Build history of the part. All positions in model axes, mm. Face numbers are marked on the shaded views. A direction names the side the tool comes from. Give positions to 0.01 mm unless a question says otherwise; leave off trailing zeros. Write each loop counter-clockwise with the first axis right and the second up, starting at its lowest first coordinate (ties: lowest second). Pieces come first, ordered by that corner, then holes. Notation, with made-up numbers: (3.5, 21.5) - (23.5, 21.5) arc R20 cw to (23.5, 59.5) - close; hole circle Ø4 at (23.5, 49). An arc over 180 degrees is marked (long way). Use one line per item in the form item = value. Start each with the question number.
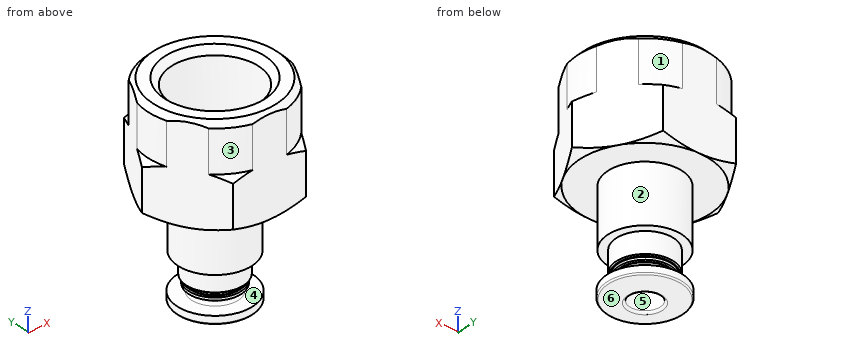
Autodesk Inventor part; units mm, degrees
ref_plane "ANBAU_STD_XY" through (0, 0, 0) normal (0, 0, -1) x (1, 0, 0)
ref_plane "ANBAU_STD_YZ" through (0, 0, 0) normal (1, 0, 0) x (0, -1, 0)
ref_plane "ANBAU_STD_ZX" through (0, 0, 0) normal (0, -1, 0) x (0, 0, -1)
sketch "Sketch_1" plane through (0, 0, 0) normal (1, 0, 0) x (0, 1, 0)
  line L0 (0, -26.9) -> (0, 0)
  line L1 (0, 0) -> (10.2, 0)
  line L2 (10.2, 0) -> (10.2, -20.6)
  line L3 (10.2, -20.6) -> (3.75, -20.6)
  line L4 (3.75, -20.6) -> (3.75, -23.35)
  line L5 (3.75, -23.35) -> (3.6, -23.5)
  line L6 (3.6, -23.5) -> (3.45, -23.5)
  line L7 (3.45, -23.5) -> (3.45, -23.85)
  line L8 (3.45, -23.85) -> (3.3, -24)
  line L9 (3.3, -24) -> (3.45, -24.15)
  line L10 (3.45, -24.15) -> (3.45, -24.5)
  line L11 (3.45, -24.5) -> (2.7, -24.5)
  line L12 (2.7, -24.5) -> (2.7, -25.05)
  arc A0 (2.7, -25.05) -> (3.05, -25.4) centre (3.05, -25.05) ccw
  line L13 (3.05, -25.4) -> (4.95, -25.4)
  line L14 (4.95, -25.4) -> (4.95, -26.2649)
  arc A1 (4.7847, -26.4619) -> (4.95, -26.2649) centre (4.75, -26.2649) ccw
  line L15 (4.7847, -26.4619) -> (2.3, -26.9)
  line L16 (2.3, -26.9) -> (0, -26.9)
  line L17 (0, -26.9) -> (0, 0)
revolve "Revolution1" add sketch "Sketch_1" angle 360 about axis through (0, 0, -26.9) along (0, 0, -1)
sketch "Sketch_2" plane through (0, 0, 0) normal (1, 0, 0) x (0, 1, 0)
  line L0 (0, -26.9) -> (0, 0)
  line L1 (0, 0) -> (6.5785, 0)
  line L2 (6.5785, 0) -> (5.7225, -0.856)
  line L3 (5.7225, -0.856) -> (5.7225, -9)
  line L4 (5.7225, -9) -> (2, -9)
  line L5 (2, -9) -> (1.5, -9.5)
  line L6 (1.5, -9.5) -> (1.5, -12)
  line L7 (1.5, -12) -> (2, -12)
  line L8 (2, -12) -> (2, -26.6)
  arc A0 (2, -26.6) -> (2.3, -26.9) centre (2.3, -26.6) ccw
  line L9 (2.3, -26.9) -> (0, -26.9)
  line L10 (0, -26.9) -> (0, 0)
revolve "Revolution2" cut sketch "Sketch_2" angle 360 about axis through (0, 0, -26.9) along (0, 0, -1)
thread "Thread1"
sketch "Sketch_3" plane through (0, 0, 0) normal (1, 0, 0) x (0, 1, 0)
  line L0 (0, -50) -> (0, 50)
  line L1 (8.5, 0) -> (10.2, -0.9815)
  line L2 (10.2, -0.9815) -> (10.2, -19.6185)
  line L3 (10.2, -19.6185) -> (8.5, -20.6)
  line L4 (8.5, -20.6) -> (13.5, -20.6)
  line L5 (13.5, -20.6) -> (13.5, 0)
  line L6 (13.5, 0) -> (8.5, 0)
revolve "Revolution3" cut sketch "Sketch_3" angle 360 about axis through (0, 0, -50) along (0, 0, -1)
sketch "Sketch_4" plane through (0, 0, 0) normal (0, 0, 1) x (1, 0, 0)
  line L0 (-17, -17) -> (17, -17)
  line L1 (17, -17) -> (17, 17)
  line L2 (17, 17) -> (-17, 17)
  line L3 (-17, 17) -> (-17, -17)
  line L4 (-9.815, 0) -> (-4.9075, -8.5)
  line L5 (-4.9075, -8.5) -> (4.9075, -8.5)
  line L6 (4.9075, -8.5) -> (9.815, 0)
  line L7 (9.815, 0) -> (4.9075, 8.5)
  line L8 (4.9075, 8.5) -> (-4.9075, 8.5)
  line L9 (-4.9075, 8.5) -> (-9.815, 0)
extrude "Extrusion1" cut sketch "Sketch_4" against normal blind 20.6
sketch "Sketch_5" plane through (0, 0, 0) normal (1, 0, 0) x (0, 1, 0)
  line L0 (0, -50) -> (0, 50)
  line L1 (8.0929, 0) -> (8.8, -0.7071)
  line L2 (8.8, -0.7071) -> (8.8, -6.1917)
  line L3 (8.8, -6.1917) -> (10.2, -7)
  line L4 (10.2, -7) -> (18.8, -7)
  line L5 (18.8, -7) -> (18.8, 0)
  line L6 (18.8, 0) -> (8.0929, 0)
revolve "Revolution4" cut sketch "Sketch_5" angle 360 about axis through (0, 0, -50) along (0, 0, -1)
sketch "Sketch_6" plane through (0, 0, 0) normal (1, 0, 0) x (0, 1, 0)
  line L0 (0, -50) -> (0, 50)
  line L1 (14.85, -9.3338) -> (8.5, -13)
  line L2 (8.5, -13) -> (4.85, -13)
  line L3 (4.85, -13) -> (4.85, -20.6)
  line L4 (4.85, -20.6) -> (14.85, -20.6)
  line L5 (14.85, -20.6) -> (14.85, -9.3338)
revolve "Revolution5" cut sketch "Sketch_6" angle 360 about axis through (0, 0, -50) along (0, 0, -1)
ref_plane "ANBAU_STD_XY" through (0, 0, 0) normal (0, 0, -1) x (1, 0, 0)
ref_plane "ANBAU_STD_YZ" through (0, 0, 0) normal (1, 0, 0) x (0, -1, 0)
ref_plane "ANBAU_STD_ZX" through (0, 0, 0) normal (0, -1, 0) x (0, 0, -1)
properties part number "190650 QSF-1/4-4-B"
(1) Cut at A-A, the plane z = -2.5. Give the cut face in (x, y) (1 decimal), then the cut area to 3 significant figures.
(2) Cut at B-B, the plane z = -15. Give the cut face in (x, y).
(3) Two-plate mould, pull along Z, no slides. Class the marked faces 4, 5 and 6: +Z half, -Z half, draft (parallel to the pull), parting line (faces both ways), or undercut.
(4) Pin check, flat tips, straight feed: pin 1 Ø6 at (y, z) = (-6, -18.5) entering from +X; pin 2 Ø4 at (y, z) = (1.5, -22) entering from +X; pin 3 Ø4 at (x, z) = (-4, -16) entering from +Y. Stop position of each tip, or through.
(5) Which spindle directions (+Z, -Z, +X, -X, +Y, -Y) get a long thin tool onto all of the face, cutting with end or side? Do the marked faces 1, 2 and 3. Say none if no direction does.
(6) Wall check: line 1 (X direction, y = 0, z = -22.75); line 2 (Z direction, x = 2.25, y = -4.25); line 3 (X direction, y = 0, z = -4.75). Give the ranges that are in metal, low to high. Write a range as from..to.
Solution:
q1.outline = (-8.5, -2.3) - (-6.2, -6.2) arc R8.8 ccw to (-2.3, -8.5) - (2.3, -8.5) arc R8.8 ccw to (6.2, -6.2) - (8.5, -2.3) arc R8.8 ccw to (8.5, 2.3) - (6.2, 6.2) arc R8.8 ccw to (2.3, 8.5) - (-2.3, 8.5) arc R8.8 ccw to (-6.2, 6.2) - (-8.5, 2.3) arc R8.8 ccw to start; hole circle Ø11.4 at (0, 0)
q1.area = 135 mm2
q2.outline = circle Ø9.7 at (0, 0); hole circle Ø4 at (0, 0)
q3.face_4 = undercut
q3.face_5 = draft
q3.face_6 = -Z half
q4.pin_1 = 3.81
q4.pin_2 = 4.85
q4.pin_3 = 4.42
q5.face_1 = +Z, +X, +Y
q5.face_2 = none
q5.face_3 = +Z, -X, -Y
q6.line_1 = -3.75..-2, 2..3.75
q6.line_2 = -26.46..-25.4, -20.6..-9
q6.line_3 = -8.8..-5.72, 5.72..8.8
